Part model, mm, in its own coordinate system. A direction names the side the tool comes from. Round coordinates to 2 decimals unless told otherwise and drop trailing zeros. Write each loop counter-clockwise with the first axis right and the second up, starting at its lowest first coordinate (ties: lowest second). Pieces come first, ordered by that corner, then holes. Notation, with made-up numbers: M -12.5,0 L 41.5,0 A23 ccw 41.5,24 Z; hole C 63.25,74 d7. An arc over 180 degrees is marked long. Answer as a JSON object with one key per item and string values. Group by question number.
1. Drill centre lines: line 1 (Z direction, x = 1.4, y = -36); line 2 (Z direction, x = 3.15, y = 27.5); line 3 (Y direction, x = 3.95, z = -120). Where is each one in solid material? Low to high. Write a range as from..to.
2. Band-saw the part on D-D, the plane y = 75. Write the cut outline in (x, z).
3. Band-saw the part on C-C, the plane z = -161. Write the cut outline in (x, y).
4. Which spindle directions (+Z, -Z, +X, -X, +Y, -Y) get a long thin tool onto all of the face, cutting with end or side? Do faces 1 (the face through (3, 36.576, -166)), 2 (the face through (2.58, 22.94, -109.3)), 3 (the face through (2.504, 50.275, -107.815)). Say none if no direction does.
5. Band-saw the part on A-A, the plane x = 3.85. Write the cut outline in (y, z), plus the area to 3 significant figures.
6. Two-plate mould, pull along Y, no slides. Class faces 4 (the face through (3, -65.024, -101)), 5 (the face through (2.576, 34.422, -103.87)), 6 (the face through (2.58, -7, -120.42)), 7 (the face through (3, -40, -31.75)): +Y half, -Y half, draft (parallel to the pull), parting line (faces both ways), or undercut.
7. Drop a flat-ended pin along its axis: pin 1 (2 mm diameter, centred on x = 1.5, z = -177, fed in from +Y). Give the stop position or say it passes through.
8. Band-saw the part on B-B, the plane y = -16.5. Write the cut outline in (x, z), plus the area to 3 significant figures.
from build123d import *

# Parameters (mm, degrees)
BOSS_EXTRUDE1_DEPTH = 5.08
CUT_EXTRUDE1_DEPTH  = 6.08
LPATTERN1_COUNT     = 2
LPATTERN1_PITCH     = 38.1
SKETCH3_W           = 5.08
SKETCH3_H           = 50.8
SKETCH3_H_2         = 101.6
CUT_EXTRUDE2_DEPTH  = 6.08


with BuildPart() as part:
    # Sketch1 → Boss-Extrude1 (new body)
    with BuildSketch(Plane(origin=(0, 0, 0), x_dir=(0, 0, -1), z_dir=(1, 0, 0))):
        Polygon((0, 0), (218.692069012, 101.977786558), (218.692069012, -65.024), (0, -65.024), align=None)
    extrude(amount=BOSS_EXTRUDE1_DEPTH)

    # Sketch2 → Cut-Extrude1 (cut, through all)
    with BuildSketch(Plane(origin=(5.08, 0, 0), x_dir=(0, 0, -1), z_dir=(1, 0, 0))):
        Polygon((101.6, 33.363958498), (106.204043558, 35.510859267), (111.571295482, 24.000750372), (106.967251924, 21.853849602), align=None)
    cut_extrude1 = extrude(amount=-CUT_EXTRUDE1_DEPTH, mode=Mode.SUBTRACT)

    # LPattern1: Cut-Extrude1 ×2
    with Locations(*[Vector(0, -0.906307787, -0.422618262) * (i * LPATTERN1_PITCH) for i in range(1, LPATTERN1_COUNT)]):
        add(cut_extrude1, mode=Mode.SUBTRACT)

    # Sketch3 → Cut-Extrude2 (cut, through all)
    with BuildSketch(Plane(origin=(5.08, 0, 0), x_dir=(0, 0, -1), z_dir=(1, 0, 0))):
        with Locations((34.29, -39.624)):
            Rectangle(SKETCH3_W, SKETCH3_H)
        with Locations((166.37, -14.224)):
            Rectangle(SKETCH3_W, SKETCH3_H_2)
    extrude(amount=-CUT_EXTRUDE2_DEPTH, mode=Mode.SUBTRACT)


solid = part.part
Worked answers:
{
 "1": {"line 1": "z = -218.69..-168.91, -163.83..-36.83, -31.75..0", "line 2": "z = -218.69..-168.91, -163.83..-109.94, -104.33..-58.97", "line 3": "y = -65.02..-6.09, -0.09..55.96"},
 "2": {"outline": "M 0,-218.69 L 5.08,-218.69 L 5.08,-160.84 L 0,-160.84 Z"},
 "3": {"outline": "M 0,-65.02 L 5.08,-65.02 L 5.08,75.08 L 0,75.08 Z"},
 "4": {"face 1": "+X, -X, -Y", "face 2": "+X, -X", "face 3": "+Z, +X, -X, +Y"},
 "5": {"outline": "M -65.02,-218.69 L 101.98,-218.69 L 0,0 L -65.02,0 L -65.02,-31.75 L -14.22,-31.75 L -14.22,-36.83 L -65.02,-36.83 L -65.02,-163.83 L 36.58,-163.83 L 36.58,-168.91 L -65.02,-168.91 Z; hole M -12.68,-123.07 L -10.53,-127.67 L 0.98,-122.31 L -1.17,-117.7 Z; hole M 21.85,-106.97 L 24,-111.57 L 35.51,-106.2 L 33.36,-101.6 Z", "area": "24,500 mm^2"},
 "6": {"face 4": "-Y half", "face 5": "undercut", "face 6": "undercut", "face 7": "draft"},
 "7": {"pin 1": "stops at y = 83"},
 "8": {"outline": "M 0,-218.69 L 5.08,-218.69 L 5.08,-168.91 L 0,-168.91 Z; M 0,-163.83 L 5.08,-163.83 L 5.08,-36.83 L 0,-36.83 Z; M 0,-31.75 L 5.08,-31.75 L 5.08,0 L 0,0 Z", "area": "1,060 mm^2"}
}
